Read the model definition and answer for the solid it produces. Units are mm, in the model's axes. A direction names the side the tool comes from. Coordinates: 2 decimals unless noted, no trailing zeros. Loops run counter-clockwise (first coordinate to the right, second up) from the corner with the lowest first, then second, coordinate; pieces in that order, holes last.
Q1. Section C-C (z = 0) is taken. Count the separate pieces of the cut face and the enclosed holes in it, then the cut area to 3 significant figures.
Q2. The mould has two halves that part along X. Classify faces 1 (the face through (58.715, -6.011, -37.17)), 2 (the face through (65.476, -6.304, 23.812)), 3 (the face through (-60.325, -6, -22)), 4 (the face through (47.02, -2.25, 1.19)): pulls with the +X half, pulls with the -X half, needs draft (parallel to the pull), parting line crosses it, or undercut.
Q3. Section A-A (x = 0) is taken. Give the vertices of the cut face in (y, z) (3 decimals), then the cut area to 3 significant figures.
Q4. Which of the six approach directions +Z, -Z, +X, -X, +Y, -Y give full straight-line access (tool end or side, diameter ignored) to faces 5 (the face through (-49.744, -6.011, 28.181)), 6 (the face through (-65.48, -5.89, 23.81)), 7 (the face through (65.5, -5.2, -20.9)), 8 (the face through (-59.04, -6.011, -36.845)), 9 (the face through (53, -4.572, -2))?
Q5. Straight lines are drawn through the part: line 1 (Z direction, x = 11, y = -5); line 2 (Z direction, x = 0, y = -9.4) (3 decimals); line 3 (X direction, y = -6, z = -24) (3 decimals). For each, find the intervals that lie inside material, in ascending order.
Q6. Section B-B (z = 31.5) is taken. Give the vertices of the cut face in (x, y) (3 decimals).
Q7. Section D-D (x = 50.8) is taken. Give the vertices of the cut face in (y, z) (3 decimals), then the cut area to 3 significant figures.
Q8. Flat-ended cylindrical pins translate along their axes: P1, Ø1.9, axis at x = 39.75, z = 42.52, coming from the +Y side; P2, Ø1.6, axis at y = -6, z = -21.5, coming from the +X side (3 decimals); P3, Ø7.5, axis at x = 50.8, z = 0, coming from the +Y side; P4, Ø1, axis at y = -5, z = -30.5, coming from the -X side (3 decimals). Find the tip coordinate at first contact, or state that the pin passes through.
from build123d import *

# Parameters (mm, degrees)
F0_R      = 2.5527
F0_R_2    = 1.5875
F0_R_3    = 2.413
F0_R_4    = 3.175
F1_DEPTH  = 12.192
F2_R      = 3.9624
F3_DEPTH  = 4.572
F4_R      = 1.6002
F5_DEPTH  = 10.16
F6_R      = 1.6002
F7_DEPTH  = 10.16
F8_R      = 2.413
F8_R_2    = 1.6002
F9_DEPTH  = 12.193
F10_R     = 4.064
F11_DEPTH = 5.08


with BuildPart() as f1:
    # F0 (on Front) → F1 (new body)
    with BuildSketch(Plane.XZ):
        Polygon((47.2694, 48.6156), (0, 48.6156), (-47.2694, 48.6156), (-70.485, 25.4), (-70.485, 0), (-70.485, -25.4), (-47.2694, -48.6156), (0, -48.6156), (47.2694, -48.6156), (70.485, -25.4), (70.485, 0), (70.485, 25.4), align=None)
        with Locations((-19.05, -42.5196)):
            Circle(F0_R, mode=Mode.SUBTRACT)
        with BuildLine():
            Line((-7.9502, -36.4236), (-40.18576, -36.4236))
            ThreePointArc((-40.18576, -36.4236), (-41.40078, -36.181918), (-42.430824, -35.493664))
            Line((-42.430824, -35.493664), (-56.855064, -21.069424))
            ThreePointArc((-56.855064, -21.069424), (-57.543318, -20.03938), (-57.785, -18.82436))
            Line((-57.785, -18.82436), (-57.785, -9.525))
            ThreePointArc((-57.785, -9.525), (-56.855064, -7.279936), (-54.61, -6.35))
            Line((-54.61, -6.35), (-7.9502, -6.35))
            ThreePointArc((-7.9502, -6.35), (-5.705136, -7.279936), (-4.7752, -9.525))
            Line((-4.7752, -9.525), (-4.7752, -33.2486))
            ThreePointArc((-4.7752, -33.2486), (-5.705136, -35.493664), (-7.9502, -36.4236))
        make_face(mode=Mode.SUBTRACT)
        with BuildLine():
            ThreePointArc((57.785, -18.82436), (57.543318, -20.03938), (56.855064, -21.069424))
            Line((56.855064, -21.069424), (42.430824, -35.493664))
            ThreePointArc((42.430824, -35.493664), (41.40078, -36.181918), (40.18576, -36.4236))
            Line((40.18576, -36.4236), (7.9502, -36.4236))
            ThreePointArc((7.9502, -36.4236), (5.705136, -35.493664), (4.7752, -33.2486))
            Line((4.7752, -33.2486), (4.7752, -9.525))
            ThreePointArc((4.7752, -9.525), (5.705136, -7.279936), (7.9502, -6.35))
            Line((7.9502, -6.35), (54.61, -6.35))
            ThreePointArc((54.61, -6.35), (56.855064, -7.279936), (57.785, -9.525))
            Line((57.785, -9.525), (57.785, -18.82436))
        make_face(mode=Mode.SUBTRACT)
        with Locations((-58.293, 0)):
            Circle(F0_R_2, mode=Mode.SUBTRACT)
        with Locations((-50.8, 0)):
            Circle(F0_R_3, mode=Mode.SUBTRACT)
        with BuildLine():
            Line((-40.18576, 36.4236), (-7.9502, 36.4236))
            ThreePointArc((-7.9502, 36.4236), (-5.705136, 35.493664), (-4.7752, 33.2486))
            Line((-4.7752, 33.2486), (-4.7752, 9.525))
            ThreePointArc((-4.7752, 9.525), (-5.705136, 7.279936), (-7.9502, 6.35))
            Line((-7.9502, 6.35), (-54.61, 6.35))
            ThreePointArc((-54.61, 6.35), (-56.855064, 7.279936), (-57.785, 9.525))
            Line((-57.785, 9.525), (-57.785, 18.82436))
            ThreePointArc((-57.785, 18.82436), (-57.543318, 20.03938), (-56.855064, 21.069424))
            Line((-56.855064, 21.069424), (-42.430824, 35.493664))
            ThreePointArc((-42.430824, 35.493664), (-41.40078, 36.181918), (-40.18576, 36.4236))
        make_face(mode=Mode.SUBTRACT)
        with Locations((-21.209, 42.5196)):
            Circle(F0_R_2, mode=Mode.SUBTRACT)
        with Locations((-13.589, 42.5196)):
            Circle(F0_R_3, mode=Mode.SUBTRACT)
        Circle(F0_R_4, mode=Mode.SUBTRACT)
        with BuildLine():
            ThreePointArc((57.785, 9.525), (56.855064, 7.279936), (54.61, 6.35))
            Line((54.61, 6.35), (7.9502, 6.35))
            ThreePointArc((7.9502, 6.35), (5.705136, 7.279936), (4.7752, 9.525))
            Line((4.7752, 9.525), (4.7752, 33.2486))
            ThreePointArc((4.7752, 33.2486), (5.705136, 35.493664), (7.9502, 36.4236))
            Line((7.9502, 36.4236), (40.18576, 36.4236))
            ThreePointArc((40.18576, 36.4236), (41.40078, 36.181918), (42.430824, 35.493664))
            Line((42.430824, 35.493664), (56.855064, 21.069424))
            ThreePointArc((56.855064, 21.069424), (57.543318, 20.03938), (57.785, 18.82436))
            Line((57.785, 18.82436), (57.785, 9.525))
        make_face(mode=Mode.SUBTRACT)
        with Locations((50.8, 0)):
            Circle(F0_R_3, mode=Mode.SUBTRACT)
        with Locations((58.293, 0)):
            Circle(F0_R_2, mode=Mode.SUBTRACT)
        with Locations((32.131, 42.5196)):
            Circle(F0_R_3, mode=Mode.SUBTRACT)
        with Locations((39.751, 42.5196)):
            Circle(F0_R_2, mode=Mode.SUBTRACT)
    extrude(amount=F1_DEPTH)

    # F2 (on face) → F3 (cut)
    with BuildSketch(Plane(origin=(0, 0, 0), x_dir=(-1, 0, 0), z_dir=(0, 1, 0))):
        with Locations((50.8, 0)):
            Circle(F2_R)
        with Locations((13.589, 42.5196)):
            Circle(F2_R)
        with Locations((-32.131, 42.5196)):
            Circle(F2_R)
        with Locations((-50.8, 0)):
            Circle(F2_R)
    extrude(amount=-F3_DEPTH, mode=Mode.SUBTRACT)

    # F4 (on face) → F5 (cut)
    with BuildSketch(Plane.YZ.offset(70.485)):
        with Locations((-6.096, 22.225)):
            Circle(F4_R)
        with Locations((-6.096, -22.225)):
            Circle(F4_R)
    extrude(amount=-F5_DEPTH, mode=Mode.SUBTRACT)

    # F6 (on face) → F7 (cut)
    with BuildSketch(Plane(origin=(-70.485, 0, 0), x_dir=(0, -1, 0), z_dir=(-1, 0, 0))):
        with Locations((6.096, 22.225)):
            Circle(F6_R)
        with Locations((6.096, -22.225)):
            Circle(F6_R)
    extrude(amount=-F7_DEPTH, mode=Mode.SUBTRACT)

    # F8 (on face) → F9 (cut, through all)
    with BuildSketch(Plane(origin=(0, 0, 0), x_dir=(-1, 0, 0), z_dir=(0, 1, 0))):
        with Locations((0, -20.32)):
            Circle(F8_R)
        with Locations((0, 20.32)):
            Circle(F8_R)
        with Locations((22.225, 0)):
            Circle(F8_R_2)
        with Locations((-22.225, 0)):
            Circle(F8_R_2)
    extrude(amount=-F9_DEPTH, mode=Mode.SUBTRACT)

    # F10 (on face) → F11 (cut)
    with BuildSketch(Plane.XZ.offset(12.192)):
        with Locations((0, -20.32)):
            Circle(F10_R)
        with Locations((0, 20.32)):
            Circle(F10_R)
    extrude(amount=-F11_DEPTH, mode=Mode.SUBTRACT)


solid = f1.part
Numbers:
1. separate pieces: 8
1. enclosed holes: 0
1. area: 1,340 mm2
2. face 1: pulls with the +X half
2. face 2: needs draft
2. face 3: pulls with the -X half
2. face 4: undercut
3. outline: (-12.192, -48.616) - (0, -48.616) - (0, -22.733) - (-7.112, -22.733) - (-7.112, -24.384) - (-12.192, -24.384) - close; (-12.192, -16.256) - (-7.112, -16.256) - (-7.112, -17.907) - (0, -17.907) - (0, -3.175) - (-12.192, -3.175) - close; (-12.192, 3.175) - (0, 3.175) - (0, 17.907) - (-7.112, 17.907) - (-7.112, 16.256) - (-12.192, 16.256) - close; (-12.192, 24.384) - (-7.112, 24.384) - (-7.112, 22.733) - (0, 22.733) - (0, 48.616) - (-12.192, 48.616) - close
3. area: 957 mm2
4. face 5: +Y, -Y
4. face 6: -X
4. face 7: +X
4. face 8: -Z, -X, +Y, -Y
4. face 9: +Y
5. line 1: z = -48.62 to -36.42, -6.35 to 6.35, 36.42 to 48.62
5. line 2: z = -48.616 to -24.384, -16.256 to -3.175, 3.175 to 16.256, 24.384 to 48.616
5. line 3: x = -70.485 to -53.924, -4.775 to 4.775, 53.924 to 70.485
6. outline: (-64.385, -12.192) - (-46.424, -12.192) - (-46.424, 0) - (-64.385, 0) - close; (-4.775, -12.192) - (4.775, -12.192) - (4.775, 0) - (-4.775, 0) - close; (46.424, -12.192) - (64.385, -12.192) - (64.385, 0) - (46.424, 0) - close
7. outline: (-12.192, -45.085) - (0, -45.085) - (0, -27.124) - (-12.192, -27.124) - close; (-12.192, -6.35) - (0, -6.35) - (0, -3.962) - (-4.572, -3.962) - (-4.572, -2.413) - (-12.192, -2.413) - close; (-12.192, 2.413) - (-4.572, 2.413) - (-4.572, 3.962) - (0, 3.962) - (0, 6.35) - (-12.192, 6.35) - close; (-12.192, 27.124) - (0, 27.124) - (0, 45.085) - (-12.192, 45.085) - close
7. area: 520 mm2
8. P1: passes through
8. P2: stops at x = 60.325
8. P3: stops at y = -4.57
8. P4: stops at x = -65.885
